from build123d import *

# Parameters (mm, degrees)
SKETCH1_W           = 81.28
SKETCH1_H           = 50.8
BOSS_EXTRUDE1_DEPTH = 1.6002
SKETCH2_R           = 1.5
CUT_EXTRUDE1_DEPTH  = 1.6002
CHAMFER1_SIZE       = 2


with BuildPart() as part:
    # Sketch1 → Boss-Extrude1 (new body)
    with BuildSketch(Plane(origin=(0, 0, 0), x_dir=(1, 0, 0), z_dir=(0, 1, 0))):
        Rectangle(SKETCH1_W, SKETCH1_H)
    extrude(amount=BOSS_EXTRUDE1_DEPTH)

    # Sketch2 → Cut-Extrude1 (cut)
    with BuildSketch(Plane(origin=(0, 1.6002, 0), x_dir=(1, 0, 0), z_dir=(0, 1, 0))):
        with Locations((-35.54, 0)):
            Circle(SKETCH2_R)
        with Locations((35.56, 0)):
            Circle(SKETCH2_R)
        Circle(SKETCH2_R)
    extrude(amount=-CUT_EXTRUDE1_DEPTH, mode=Mode.SUBTRACT)

    # Chamfer1
    chamfer1_edges = [part.edges().sort_by_distance(p)[0] for p in [
        (40.64, 0.8001, 25.4),
        (-40.64, 0.8001, 25.4),
        (-40.64, 0.8001, -25.4),
        (40.64, 0.8001, -25.4),
    ]]
    chamfer(chamfer1_edges, length=CHAMFER1_SIZE)


solid = part.part
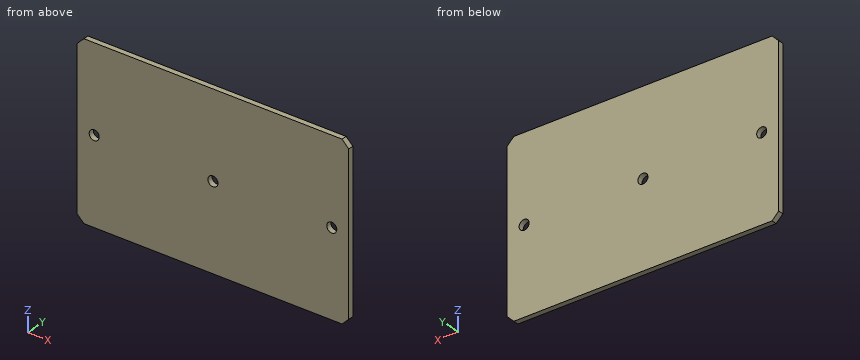
Can you work these out from the model? Positions are in its coordinate system, mm. Coordinates: 2 decimals unless noted, no trailing zeros. Write each loop counter-clockwise with the first axis right and the second up, starting at its lowest first coordinate (ties: lowest second). Pieces come first, ordered by that corner, then holes. Notation, with made-up numbers: (81.25, 72) - (125.25, 72) arc R21 cw to (125.25, 89) - close; hole circle Ø8 at (68.5, 0.25). An arc over 180 degrees is marked (long way). Return JSON: item names as keys, results as strings. Group by question number.
Item 1: Please list where these lines run through material, in increasing order: probe 1 along X at (y, z) = (0.45, 0); probe 2 along Z at (x, y) = (-35.54, 0.7); probe 3 along Z at (x, y) = (0.5, 1.15).
Item 2: I'm going to push a flat-ended pin straight in: pin 1 Ø2.5 at (x, z) = (0, 0) entering from -Y. Where does the tip first touch, or does it pass through?
Item 3: If we section it at B-B (x = 0): Write out the boundary of the cut face in (y, z), then the cut area to 3 significant figures.
Item 4: If we section it at A-A (z = 0): Write out the boundary of the cut face in (x, y).
Return value:
{
 "1": {"probe 1": "x = -40.64 to -37.04, -34.04 to -1.5, 1.5 to 34.06, 37.06 to 40.64", "probe 2": "z = -25.4 to -1.5, 1.5 to 25.4", "probe 3": "z = -25.4 to -1.41, 1.41 to 25.4"},
 "2": {"pin 1": "passes through"},
 "3": {"outline": "(0, -25.4) - (1.6, -25.4) - (1.6, -1.5) - (0, -1.5) - close; (0, 1.5) - (1.6, 1.5) - (1.6, 25.4) - (0, 25.4) - close", "area": "76.5 mm^2"},
 "4": {"outline": "(-40.64, 0) - (-37.04, 0) - (-37.04, 1.6) - (-40.64, 1.6) - close; (-34.04, 0) - (-1.5, 0) - (-1.5, 1.6) - (-34.04, 1.6) - close; (1.5, 0) - (34.06, 0) - (34.06, 1.6) - (1.5, 1.6) - close; (37.06, 0) - (40.64, 0) - (40.64, 1.6) - (37.06, 1.6) - close"}
}
